For this review, take the finished solid that the model builds, in its own axes (mm). Give positions to 0.01 mm unless a question says otherwise; leave off trailing zeros. Order: outer loops, then holes, each group sorted by start corner. A loop starts at its lowest first (then second) coordinate and runs counter-clockwise, first axis right, second up. Notation, with made-up numbers: (80.25, 2) -> (104.25, 2) arc R14 cw to (104.25, 22) -> close; hole circle Ø11 at (54, 33). An arc over 180 degrees is marked (long way). Return JSON: item names as keys, results as strings. Group by question number.
1) Add section A-A (x = 0). Give the boundary of the cut face in (y, z) (3 decimals), then the cut area to 3 significant figures.
2) Add section B-B (z = 2.4). Give the boundary of the cut face in (x, y), then the cut area to 3 significant figures.
3) Insertion check: P1, Ø14.5, axis at x = 0, y = -10.2, coming from the +Z side (3 decimals); P2, Ø7.5, axis at x = 0, y = 15.2, coming from the -Z side. Each pin has a flat end and moves straight along its axis. Give the tip position at first contact, or say it passes through.
4) To check wall thickness, follow line 1 along X through (y, z) = (13.5, 1.75); line 2 along X through (y, z) = (-14, 1.7). State the ranges of each line that lie inside material, in increasing order.
5) The part is to be moulded in two halves that separate along X. For faces 1 (the face through (-12.7, -1, 2)), 2 (the face through (0.8, -41.9, 1.6)), 3 (the face through (12.7, -1, 2)), say which applies: released by +X, released by -X, zero draft, split by the parting line, or undercut.
from build123d import *

# Parameters (mm, degrees)
F0_W     = 25.4
F0_H     = 152.4
F1_DEPTH = 3.175
F3_D     = 12.7
F3_DEPTH = 25.4
F3_TIP   = 3.8154649308
F4_D     = 12.7
F4_DEPTH = 25.4
F4_TIP   = 3.8154649308


with BuildPart() as f1:
    # F0 (on Top) → F1 (new body)
    with BuildSketch(Plane.XY):
        Rectangle(F0_W, F0_H)
    extrude(amount=F1_DEPTH)

    # F3
    with Locations(Plane(origin=(0, 0, 0), x_dir=(1, 0, 0), z_dir=(0, 0, -1))):
        with Locations((0, 61.0016693357)):
            Hole(F3_D / 2, depth=F3_DEPTH)
            with Locations((0, 0, -(F3_DEPTH + F3_TIP / 2))):  # 118° drill point
                Cone(0, F3_D / 2, F3_TIP, mode=Mode.SUBTRACT)

    # F4
    with Locations(Plane(origin=(0, 0, 0), x_dir=(1, 0, 0), z_dir=(0, 0, -1))):
        with Locations((0, 35.6016693357), (0, 10.2016693357), (0, -15.1983306643), (0, -40.5983306643), (0, -65.9983306643), (0, -91.3983306643), (0, -116.7983306643), (0, -142.1983306643)):
            Hole(F4_D / 2, depth=F4_DEPTH)
            with Locations((0, 0, -(F4_DEPTH + F4_TIP / 2))):  # 118° drill point
                Cone(0, F4_D / 2, F4_TIP, mode=Mode.SUBTRACT)


solid = f1.part
Evaluation:
{
 "1": {"outline": "(-76.2, 0) -> (-67.352, 0) -> (-67.352, 3.175) -> (-76.2, 3.175) -> close; (-54.652, 0) -> (-41.952, 0) -> (-41.952, 3.175) -> (-54.652, 3.175) -> close; (-29.252, 0) -> (-16.552, 0) -> (-16.552, 3.175) -> (-29.252, 3.175) -> close; (-3.852, 0) -> (8.848, 0) -> (8.848, 3.175) -> (-3.852, 3.175) -> close; (21.548, 0) -> (34.248, 0) -> (34.248, 3.175) -> (21.548, 3.175) -> close; (46.948, 0) -> (59.648, 0) -> (59.648, 3.175) -> (46.948, 3.175) -> close; (72.348, 0) -> (76.2, 0) -> (76.2, 3.175) -> (72.348, 3.175) -> close", "area": "242 mm^2"},
 "2": {"outline": "(-12.7, -76.2) -> (12.7, -76.2) -> (12.7, 76.2) -> (-12.7, 76.2) -> close; hole circle Ø12.7 at (0, -61); hole circle Ø12.7 at (0, -35.6); hole circle Ø12.7 at (0, -10.2); hole circle Ø12.7 at (0, 15.2); hole circle Ø12.7 at (0, 40.6); hole circle Ø12.7 at (0, 66)", "area": "3,110 mm^2"},
 "3": {"P1": "z = 3.175", "P2": "through"},
 "4": {"line 1": "-12.7 to -6.12, 6.12 to 12.7", "line 2": "-12.7 to -5.09, 5.09 to 12.7"},
 "5": {"face 1": "released by -X", "face 2": "undercut", "face 3": "released by +X"}
}
